Could you check a few things on this model? Use its own coordinates, in mm. Face numbers are marked on the shaded views. Give positions to 0.01 mm unless a question says otherwise; leave off trailing zeros. Loops run counter-clockwise (first coordinate to the right, second up) from the corner with the lowest first, then second, coordinate; pieces in that order, holes last. Notation, with made-up numbers: (-39, 81) - (-26, 81) arc R16 cw to (-26, 111) - close; hole circle Ø8 at (-9, 21.25). An arc over 180 degrees is marked (long way). One line per item, written item: value. Start each with the question number.
Q1. If we mould it in two halves opening along X, with no side actions, what happens to the marked faces 1, 2, 3 and 4? For each: released by +X, released by -X, zero draft, split by the parting line, or undercut.
Q2. I want a section at B-B (x = 0). Please give me the cut outline in (y, z) (3 decimals), then the cut area to 3 significant figures.
Q3. I want a section at D-D (z = 39). Please give me the cut outline in (x, y), then the cut area to 3 significant figures.
Q4. I want a section at A-A (y = -13). Please give me the cut outline in (x, z), then the cut area to 3 significant figures.
Q5. If I drill on line 1 (Y direction, x = 0, z = 37.15) (3 decimals); line 2 (Z direction, x = 0.25, y = -7); line 3 (X direction, y = 33, z = 47.75), over which ranges is the centre line in solid material (lowest first)? Write a range as from..to.
Q6. I'm going to push flat-ended pins straight in: P1, Ø10, axis at x = 3, y = 10.5, coming from the -Z side; P2, Ø4, axis at x = -9.5, z = 40.5, coming from the +Y side; P3, Ø2, axis at x = 10, z = 39.5, coming from the +Y side. Where does each tip first touch, or does it pass through?
Q7. I want a section at C-C (z = 45.25). Please give me the cut outline in (x, y).
```python
from build123d import *

# Parameters (mm, degrees)
F0_W     = 101.6
F0_H     = 101.6
F1_DEPTH = 50.8
F3_DEPTH = 12.7
F4_R     = 7.62
F4_R_2   = 6.985
F5_DEPTH = 1.27
F6_SIZE  = 0.762
F7_R     = 0.762
F9_DEPTH = 25.4
F10_R    = 2.54


with BuildPart() as f1:
    # F0 (on Top) → F1 (new body)
    with BuildSketch(Plane.XY):
        Rectangle(F0_W, F0_H)
    extrude(amount=F1_DEPTH)

    # F2 (on face) → F3 (cut)
    with BuildSketch(Plane.XY.offset(50.8)):
        with BuildLine():
            Line((-12.7, 25.4), (12.7, 25.4))
            ThreePointArc((12.7, 25.4), (0, 38.1), (-12.7, 25.4))
        make_face()
        with BuildLine():
            ThreePointArc((-12.7, 25.4), (0, 12.7), (12.7, 25.4))
            Line((12.7, 25.4), (-12.7, 25.4))
        make_face()
        with BuildLine():
            ThreePointArc((-12.7, -25.4), (0, -12.7), (12.7, -25.4))
            Line((12.7, -25.4), (12.7, 25.4))
            ThreePointArc((12.7, 25.4), (0, 12.7), (-12.7, 25.4))
            Line((-12.7, 25.4), (-12.7, -25.4))
        make_face()
        with BuildLine():
            Line((-12.7, -25.4), (12.7, -25.4))
            ThreePointArc((12.7, -25.4), (0, -12.7), (-12.7, -25.4))
        make_face()
        with BuildLine():
            ThreePointArc((-12.7, -25.4), (0, -38.1), (12.7, -25.4))
            Line((12.7, -25.4), (-12.7, -25.4))
        make_face()
    extrude(amount=-F3_DEPTH, mode=Mode.SUBTRACT)

    # F4 (on face) → F5 (cut)
    with BuildSketch(Plane.XY.offset(38.1)):
        with Locations((0, -25.4)):
            Circle(F4_R)
        with Locations((0, -25.4)):
            Circle(F4_R_2, mode=Mode.SUBTRACT)
    extrude(amount=-F5_DEPTH, mode=Mode.SUBTRACT)

    # F6
    f6_edges = [f1.edges().sort_by_distance(p)[0] for p in [
        (-7.62, -25.4, 38.1),
        (0, -50.8, 0),
    ]]
    chamfer(f6_edges, length=F6_SIZE)

    # F7
    f7_edges = [f1.edges().sort_by_distance(p)[0] for p in [
        (-6.985, -25.4, 38.1),
    ]]
    fillet(f7_edges, radius=F7_R)

    # F10
    f10_edges = [f1.edges().sort_by_distance(p)[0] for p in [
        (0, -38.1, 38.1),
    ]]
    fillet(f10_edges, radius=F10_R)


with BuildPart() as f9:
    # F8 (on face) → F9 (new body)
    with BuildSketch(Plane.XY.offset(50.8)):
        with BuildLine():
            ThreePointArc((-12.7, -25.4), (0, -38.1), (12.7, -25.4))
            Line((12.7, -25.4), (12.7, 25.4))
            ThreePointArc((12.7, 25.4), (0, 38.1), (-12.7, 25.4))
            Line((-12.7, 25.4), (-12.7, -25.4))
        make_face()
    extrude(amount=-F9_DEPTH)

    # F11: cut F1
    add(f1.part, mode=Mode.SUBTRACT)


solid = f9.part
```
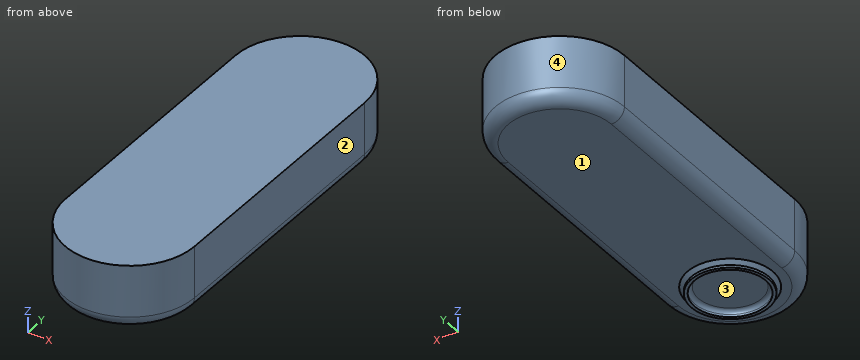
Worked answers:
1. face 1: zero draft
1. face 2: released by +X
1. face 3: undercut
1. face 4: split by the parting line
2. outline: (-38.1, 40.64) arc R2.54 ccw to (-35.56, 38.1) - (-33.782, 38.1) - (-33.02, 37.338) - (-33.02, 36.83) - (-32.385, 36.83) - (-32.385, 37.338) arc R0.762 cw to (-31.623, 38.1) - (-19.177, 38.1) arc R0.762 cw to (-18.415, 37.338) - (-18.415, 36.83) - (-17.78, 36.83) - (-17.78, 37.338) - (-17.018, 38.1) - (35.56, 38.1) arc R2.54 ccw to (38.1, 40.64) - (38.1, 50.8) - (-38.1, 50.8) - close
2. area: 967 mm²
3. outline: (-12.1, -25.4) arc R12.1 ccw to (12.1, -25.4) - (12.1, 25.4) arc R12.1 ccw to (-12.1, 25.4) - close
3. area: 1,690 mm²
4. outline: (-12.7, 40.64) arc R2.54 ccw to (-10.16, 38.1) - (10.16, 38.1) arc R2.54 ccw to (12.7, 40.64) - (12.7, 50.8) - (-12.7, 50.8) - close
4. area: 320 mm²
5. line 1: y = -33.02..-32.385, -18.415..-17.78
5. line 2: z = 38.1..50.8
5. line 3: x = -10.17..10.17
6. P1: stops at z = 38.1
6. P2: stops at y = 35.65
6. P3: stops at y = 34.12
7. outline: (-12.7, -25.4) arc R12.7 ccw to (12.7, -25.4) - (12.7, 25.4) arc R12.7 ccw to (-12.7, 25.4) - close
